from build123d import *

# Parameters (mm, degrees)
BOSS_EXTRUDE1_DEPTH  = 19.05
SKETCH3_R            = 1.4986
CUT_EXTRUDE1_DEPTH   = 52.081415314
BOSS_EXTRUDE2_DEPTH  = 2.9972
SKETCH5_W            = 2.9972
SKETCH5_H            = 6.35
BOSS_EXTRUDE3_DEPTH  = 2.9972
FILLET1_R            = 0.635
FILLET1_OF_MIRROR1_R = 0.635


with BuildPart() as part:
    # Sketch1 → Revolve1 (revolve)
    with BuildSketch(Plane.XY, mode=Mode.PRIVATE) as revolve1_sk:
        Polygon((-4, -19.7), (0, -19.7), (0, 19.7), (-4, 19.7), (-4, 12.7), (-7.9375, 12.7), (-7.9375, 9.525), (-12.7, 9.525), (-12.7, -9.525), (-7.9375, -9.525), (-7.9375, -12.7), (-4, -12.7), align=None)
    revolve(revolve1_sk.sketch.rotate(Axis((0, 0, 0), (0, 1, 0)), 180), axis=Axis((0, 0, 0), (0, 1, 0)))

    # Sketch2 → Boss-Extrude1 (add)
    with BuildSketch(Plane(origin=(0, 9.525, 0), x_dir=(1, 0, 0), z_dir=(0, 1, 0))):
        Polygon((12.7, 0), (23.672555951, 9.207067652), (12.7, 22.283650626), (-12.7, 22.283650626), (-12.7, 0), align=None)
    extrude(amount=-BOSS_EXTRUDE1_DEPTH)

    # Sketch3 → Cut-Extrude1 (cut, through all)
    with BuildSketch(Plane(origin=(0, 19.7, 0), x_dir=(1, 0, 0), z_dir=(0, 1, 0))):
        with Locations(Location((0, 0, 0), (0, 0, 180))):
            Circle(SKETCH3_R)
    extrude(amount=-CUT_EXTRUDE1_DEPTH, mode=Mode.SUBTRACT)

    # Sketch4 → Boss-Extrude2 (add)
    with BuildSketch(Plane(origin=(0, 9.525, 0), x_dir=(1, 0, 0), z_dir=(0, 1, 0))):
        Polygon((15.779368843, 15.017901691), (13.483380438, 13.091338668), (17.56508176, 8.226956454), (19.861070165, 10.153519478), align=None)
    boss_extrude2 = extrude(amount=BOSS_EXTRUDE2_DEPTH)

    # Sketch5 → Boss-Extrude3 (add)
    with BuildSketch(Plane(origin=(0, 9.525, 0), x_dir=(1, 0, 0), z_dir=(0, 1, 0))):
        with Locations((-8.89, 19.057850626)):
            Rectangle(SKETCH5_W, SKETCH5_H)
        with Locations((8.89, 19.057850626)):
            Rectangle(SKETCH5_W, SKETCH5_H)
    boss_extrude3 = extrude(amount=BOSS_EXTRUDE3_DEPTH)

    # Fillet1
    fillet1_edges = [part.edges().sort_by_distance(p)[0] for p in [
        (-7.3914, 12.5222, -19.057850626),
        (-8.89, 12.5222, -22.232850626),
        (-10.3886, 12.5222, -19.057850626),
        (-8.89, 12.5222, -15.882850626),
        (10.3886, 12.5222, -19.057850626),
        (8.89, 12.5222, -22.232850626),
        (7.3914, 12.5222, -19.057850626),
        (8.89, 12.5222, -15.882850626),
        (17.820219504, 12.5222, -12.585710584),
        (14.631374641, 12.5222, -14.054620179),
        (15.524231099, 12.5222, -10.659147561),
        (18.713075962, 12.5222, -9.190237966),
    ]]
    fillet(fillet1_edges, radius=FILLET1_R)

    # Mirror1: Boss-Extrude2, Boss-Extrude3 across plane
    add(boss_extrude2.mirror(Plane.ZX))
    add(boss_extrude3.mirror(Plane.ZX))

    # Fillet1 of Mirror1
    fillet1_of_mirror1_edges = [part.edges().sort_by_distance(p)[0] for p in [
        (-7.3914, -12.5222, -19.057850626),
        (-8.89, -12.5222, -22.232850626),
        (-10.3886, -12.5222, -19.057850626),
        (-8.89, -12.5222, -15.882850626),
        (10.3886, -12.5222, -19.057850626),
        (8.89, -12.5222, -22.232850626),
        (7.3914, -12.5222, -19.057850626),
        (8.89, -12.5222, -15.882850626),
        (17.820219504, -12.5222, -12.585710584),
        (14.631374641, -12.5222, -14.054620179),
        (15.524231099, -12.5222, -10.659147561),
        (18.713075962, -12.5222, -9.190237966),
    ]]
    fillet(fillet1_of_mirror1_edges, radius=FILLET1_OF_MIRROR1_R)


solid = part.part
Model file for the job. Use its own axes, mm. A direction names the side the tool comes from. Give positions to 0.01 mm unless a question says otherwise; leave off trailing zeros. Loops run counter-clockwise (first coordinate to the right, second up) from the corner with the lowest first, then second, coordinate; pieces in that order, holes last.
Item 1: Slice it at C-C (z = 7). Write the cut outline in (x, y) (3 decimals), plus the area to 3 significant figures.
Check values:
outline: (-10.597, -9.525) - (-3.742, -9.525) - (-3.742, -12.7) - (3.742, -12.7) - (3.742, -9.525) - (10.597, -9.525) - (10.597, 9.525) - (3.742, 9.525) - (3.742, 12.7) - (-3.742, 12.7) - (-3.742, 9.525) - (-10.597, 9.525) - close
area: 451 mm2
Item 2: Mould opens along Z. For faces 5 (the face through (-1.72, -11.13, 7.75)), 6 (the face through (9, 11, -22.233)), 7 (the face through (17, -12.522, -12)) say: +Z half, -Z half, draft (parallel to the pull), parting line (faces both ways), or undercut.
Check values:
face 5: undercut
face 6: -Z half
face 7: draft
Item 3: Slice it at A-A (y = 8.5). Write the cut outline in (x, z).
Check values:
outline: (-12.7, -22.28) - (12.7, -22.28) - (23.67, -9.21) - (12.7, 0) arc R12.7 ccw to (-12.7, 0) - close; hole circle Ø3 at (0, 0)
Item 4: Which spindle directions (+Z, -Z, +X, -X, +Y, -Y) get a long thin tool onto all of the face, cutting with end or side? Do faces 1 (the face through (-0.867, -16.249, 3.905)), 2 (the face through (-9, 11, -15.883)), 3 (the face through (-9, -11, -22.233)), 4 (the face through (-1.72, 11.09, 7.75)). Say none if no direction does.
Check values:
face 1: -Y
face 2: +X, -X, +Y
face 3: -Z, +X, -X, -Y
face 4: +Y
Item 5: Drop flat-ended pins along their axis: P1, Ø1.2, axis at y = 10.5, z = -19, coming from the +X side; P2, Ø0.7, axis at x = -9, y = 10.5, coming from the +Z side; P3, Ø1, axis at x = 7, z = -12.5, coming from the -Y side (3 decimals). Give the stop position or say it passes through.
Check values:
P1: stops at x = 10.39
P2: stops at z = -15.88
P3: stops at y = -9.525
Item 6: Slice it at B-B (x = 0). Write the cut outline in (y, z) (1 decimal).
Check values:
outline: (-19.7, -4) - (-12.7, -4) - (-12.7, -7.9) - (-9.5, -7.9) - (-9.5, -22.3) - (9.5, -22.3) - (9.5, -7.9) - (12.7, -7.9) - (12.7, -4) - (19.7, -4) - (19.7, -1.5) - (-19.7, -1.5) - close; (-19.7, 1.5) - (19.7, 1.5) - (19.7, 4) - (12.7, 4) - (12.7, 7.9) - (9.5, 7.9) - (9.5, 12.7) - (-9.5, 12.7) - (-9.5, 7.9) - (-12.7, 7.9) - (-12.7, 4) - (-19.7, 4) - close
Item 7: Slice it at D-D (y = -14.5). Write the cut outline in (x, z), plus the area to 3 significant figures.
Check values:
outline: circle Ø8 at (0, 0); hole circle Ø3 at (0, 0)
area: 43.2 mm2
Item 8: Drill centre lines: line 1 along Z through (x, y) = (0, 9); line 2 along Y through (x, z) = (18, -5.5) (3 decimals); line 3 along Y through (x, z) = (9, -17). Where is each one in solid material? Low to high.
Check values:
line 1: z = -22.28 to -1.5, 1.5 to 12.7
line 2: y = -9.525 to 9.525
line 3: y = -12.52 to 12.52
